Here's how the part is built. I have some questions about the finished solid (model axes, mm). A direction names the side the tool comes from. Coordinates: 2 decimals unless noted, no trailing zeros. Write each loop counter-clockwise with the first axis right and the second up, starting at its lowest first coordinate (ties: lowest second). Pieces come first, ordered by that corner, then holes.
```python
from build123d import *

# Parameters (mm, degrees)
SKETCH1_R           = 11.5
BOSS_EXTRUDE1_DEPTH = 66
SKETCH2_R           = 1.5
BOSS_EXTRUDE2_DEPTH = 10
BOSS_EXTRUDE4_START = 6
SKETCH4_R           = 1.5
BOSS_EXTRUDE4_DEPTH = 6
FILLET1_R           = 0.5
CUT_EXTRUDE1_START  = -5
CUT_EXTRUDE1_DEPTH  = 5


with BuildPart() as part:
    # Sketch1 → Boss-Extrude1 (new body)
    with BuildSketch(Plane(origin=(0, 0, 0), x_dir=(1, 0, 0), z_dir=(0, 1, 0))):
        with Locations(Location((0, 0, 0), (0, 0, 270))):
            Circle(SKETCH1_R)
    extrude(amount=BOSS_EXTRUDE1_DEPTH)

    # Sketch2 → Boss-Extrude2 (add)
    with BuildSketch(Plane(origin=(0, 66, 0), x_dir=(1, 0, 0), z_dir=(0, 1, 0))):
        with Locations(Location((0, 0, 0), (0, 0, 270))):
            Circle(SKETCH2_R)
    extrude(amount=BOSS_EXTRUDE2_DEPTH)

    # Sketch4 → Boss-Extrude4 (add)
    with BuildSketch(Plane.XZ.offset(BOSS_EXTRUDE4_START)):
        with Locations(Location((0, 0, 0), (0, 0, 90))):
            Circle(SKETCH4_R)
    extrude(amount=-BOSS_EXTRUDE4_DEPTH)

    # Fillet1
    fillet1_edges = [part.edges().sort_by_distance(p)[0] for p in [
        (0, -6, -1.5),
    ]]
    fillet(fillet1_edges, radius=FILLET1_R)

    # Sketch5 → Cut-Extrude1 (cut)
    with BuildSketch(Plane(origin=(0, 76, 0), x_dir=(1, 0, 0), z_dir=(0, 1, 0)).offset(CUT_EXTRUDE1_START)):
        with BuildLine():
            Line((0.765599936, 1.289905709), (0.765599936, -1.289905709))
            ThreePointArc((0.765599936, -1.289905709), (1.5, 0), (0.765599936, 1.289905709))
        make_face()
    extrude(amount=CUT_EXTRUDE1_DEPTH, mode=Mode.SUBTRACT)


solid = part.part
```
1) I need wall thicknesses on probe 1 along Y at (x, z) = (-6.5, 3); probe 2 along X at (y, z) = (40, -0.25); probe 3 along Z at (x, y) = (-3.5, 7.5). Which ranges of each line are inside material? Lowest first, please.
Values follow:
probe 1: y = 0 to 66
probe 2: x = -11.5 to 11.5
probe 3: z = -10.95 to 10.95
2) On a 3-axis mill with a long thin cutter (end or side, diameter ignored), from which of +Z, -Z, +X, -X, +Y, -Y can I reach the whole of each face in a straight line? I mean faces 1 (the face through (-1.33, 70.93, 0.69)), 2 (the face through (-0.45, -2.79, 1.43)), 3 (the face through (0, 76, 0)), 4 (the face through (0.766, 73, 0)). Say none if no direction works.
Values follow:
face 1: +Y
face 2: -Y
face 3: +Z, -Z, +X, -X, +Y
face 4: +Z, -Z, +X, +Y
3) Imagine slicing it at A-A on z = 0. Please give me the cut outline in (x, y), then the cut area to 3 significant figures.
Values follow:
outline: (-11.5, 0) - (-1.5, 0) - (-1.5, -5.5) arc R0.5 ccw to (-1, -6) - (1, -6) arc R0.5 ccw to (1.5, -5.5) - (1.5, 0) - (11.5, 0) - (11.5, 66) - (1.5, 66) - (1.5, 71) - (0.77, 71) - (0.77, 76) - (-1.5, 76) - (-1.5, 66) - (-11.5, 66) - close
area: 1,560 mm2
4) Imagine slicing it at B-B on x = 0. Please give me the cut outline in (y, z).
Values follow:
outline: (-6, -1) arc R0.5 ccw to (-5.5, -1.5) - (0, -1.5) - (0, -11.5) - (66, -11.5) - (66, -1.5) - (76, -1.5) - (76, 1.5) - (66, 1.5) - (66, 11.5) - (0, 11.5) - (0, 1.5) - (-5.5, 1.5) arc R0.5 ccw to (-6, 1) - close
5) Imagine slicing it at C-C on y = 43.5. Please give me the cut outline in (x, z).
Values follow:
outline: circle Ø23 at (0, 0)
6) Imagine slicing it at D-D on z = -4.25. Please give me the cut outline in (x, y), then the cut area to 3 significant figures.
Values follow:
outline: (-10.69, 0) - (10.69, 0) - (10.69, 66) - (-10.69, 66) - close
area: 1,410 mm2
7) Will these pins go through, and if not, where does the flat tip stop? pin 1 (1 mm diameter, centred on x = -5, y = 27.5, fed in from +Z); pin 2 (6 mm diameter, centred on x = 8.5, y = 51.5, fed in from +Z); pin 3 (12 mm diameter, centred on y = 64.5, z = 7, fed in from +X).
Values follow:
pin 1: stops at z = 10.58
pin 2: stops at z = 10.1
pin 3: stops at x = 11.46
